Here's how the part is built. I have some questions about the finished solid (model axes, mm). Face numbers are marked on the shaded views. A direction names the side the tool comes from. Coordinates: 2 decimals unless noted, no trailing zeros. Loops run counter-clockwise (first coordinate to the right, second up) from the corner with the lowest first, then second, coordinate; pieces in that order, holes last. Notation, with made-up numbers: (-33.5, 43) -> (16.5, 43) arc R28 cw to (16.5, 75) -> close; hole circle Ø10 at (74.25, -0.5). An arc over 180 degrees is marked (long way). Answer as a JSON object with one key per item and string values. Group by question number.
Q1. I want a section at A-A on y = 3.5. Count the separate pieces of the cut face and the enclosed holes in it, then the cut area to 3 significant figures.
Q2. On a 3-axis mill with a long thin cutter (end or side, diameter ignored), from which of +Z, -Z, +X, -X, +Y, -Y can I reach the whole of each face in a straight line? I mean the marked faces 5, 6, 7 and 8. Say none if no direction works.
Q3. Thinking about a two-plate mould opening in Z: for the marked faces 1, 2, 3 and 4, which applies, released by +Z, released by -Z, zero draft, split by the parting line, or undercut?
Q4. I want a section at D-D on z = -9.5. Write out the boundary of the cut face in (x, y), then the cut area to 3 significant figures.
Q5. I need wall thicknesses on line 1 (X direction, y = 0.5, z = -13); line 2 (X direction, y = 1, z = -1.25); line 3 (Y direction, x = -3, z = 1). Which ranges of each line are inside material? Lowest first, please.
Q6. I'm going to push flat-ended pins straight in: pin 1 (2.5 mm diameter, centred on y = 5.5, z = -13, fed in from -X); pin 2 (1.5 mm diameter, centred on x = -10, z = -6, fed in from +Y); pin 3 (4 mm diameter, centred on y = 3, z = -14, fed in from +X). Where does each tip first touch, or does it pass through?
Q7. I want a section at B-B on z = -1.75. Write out the boundary of the cut face in (x, y), then the cut area to 3 significant figures.
Q8. I want a section at C-C on x = -12. Write out the boundary of the cut face in (y, z) (3 decimals).
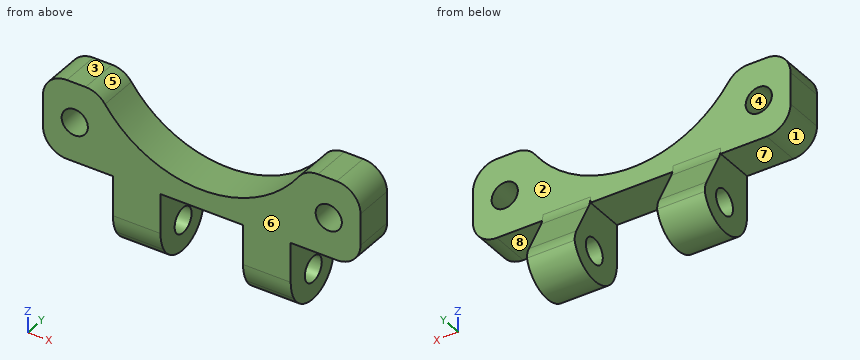
```python
from build123d import *

# Parameters (mm, degrees)
ESQUISSE1_W                    = 40
ESQUISSE1_H                    = 10
BOSS_EXTRU_1_DEPTH             = 5
ESQUISSE2_R                    = 1.65
ENL_V_MAT_EXTRU_1_DEPTH        = 5
BOSS_EXTRU_2_REACH             = 41.929
ESQUISSE3_W                    = 6
ESQUISSE3_H                    = 10
BOSS_EXTRU_2_DIRECTION_2_DEPTH = 5
ESQUISSE4_R                    = 1.6
ENL_V_MAT_EXTRU_2_DEPTH        = 38.217801601
CONG_1_R                       = 5
ENL_V_MAT_EXTRU_3_DEPTH        = 38.217801601
CONG_3_R                       = 3
CONG_4_R                       = 3
CONG_5_R                       = 3
ENL_V_MAT_EXTRU_4_REACH        = 44.982
CONG_6_R                       = 3
CONG_7_START                   = -30.067545716
CONG_7_DEPTH                   = 22.4


with BuildPart() as part:
    # Esquisse1 → Boss.-Extru.1 (new body)
    with BuildSketch(Plane(origin=(0, 0, 0), x_dir=(1, 0, 0), z_dir=(0, 1, 0))):
        with Locations((-18.867545716, 2.655728702)):
            Rectangle(ESQUISSE1_W, ESQUISSE1_H)
    extrude(amount=BOSS_EXTRU_1_DEPTH)

    # Esquisse2 → Enlèv. mat.-Extru.1 (cut)
    with BuildSketch(Plane(origin=(0, 5, 0), x_dir=(1, 0, 0), z_dir=(0, 1, 0))):
        with Locations(Location((-34.867545716, 2.655728702, 0), (0, 0, 270))):
            Circle(ESQUISSE2_R)
        with Locations(Location((-2.867545716, 2.655728702, 0), (0, 0, 270))):
            Circle(ESQUISSE2_R)
    extrude(amount=-ENL_V_MAT_EXTRU_1_DEPTH, mode=Mode.SUBTRACT)

    # Boss.-Extru.2: up to this face of the body (flat: up to its plane)
    boss_extru_2_end = Plane(part.part.faces().sort_by_distance((-18.867545716, 0, -2.655728702))[0])
    # Esquisse3 → Boss.-Extru.2 (add, up to the picked face)
    with BuildSketch(Plane(origin=(0, 5, 0), x_dir=(1, 0, 0), z_dir=(0, 1, 0)), mode=Mode.PRIVATE) as boss_extru_2_sk1:
        with Locations((-10.667545716, 12.655728702)):
            Rectangle(ESQUISSE3_W, ESQUISSE3_H)
    boss_extru_2_tool1 = split(extrude(boss_extru_2_sk1.sketch, amount=-BOSS_EXTRU_2_REACH, mode=Mode.PRIVATE), bisect_by=boss_extru_2_end, keep=Keep.BOTH, mode=Mode.PRIVATE)
    # Esquisse3 → Boss.-Extru.2 (add, up to the picked face)
    with BuildSketch(Plane(origin=(0, 5, 0), x_dir=(1, 0, 0), z_dir=(0, 1, 0)), mode=Mode.PRIVATE) as boss_extru_2_sk2:
        with Locations((-27.067545716, 12.655728702)):
            Rectangle(ESQUISSE3_W, ESQUISSE3_H)
    boss_extru_2_tool2 = split(extrude(boss_extru_2_sk2.sketch, amount=-BOSS_EXTRU_2_REACH, mode=Mode.PRIVATE), bisect_by=boss_extru_2_end, keep=Keep.BOTH, mode=Mode.PRIVATE)
    add(boss_extru_2_tool1.solids().sort_by(Axis((-10.667546, 5, -12.655729), (0, -1, 0)))[0])
    add(boss_extru_2_tool2.solids().sort_by(Axis((-27.067546, 5, -12.655729), (0, -1, 0)))[0])

    # Esquisse3 → Boss.-Extru.2 direction 2 (add)
    with BuildSketch(Plane(origin=(0, 5, 0), x_dir=(1, 0, 0), z_dir=(0, 1, 0))):
        with Locations((-10.667545716, 12.655728702)):
            Rectangle(ESQUISSE3_W, ESQUISSE3_H)
        with Locations((-27.067545716, 12.655728702)):
            Rectangle(ESQUISSE3_W, ESQUISSE3_H)
    extrude(amount=BOSS_EXTRU_2_DIRECTION_2_DEPTH)

    # Esquisse4 → Enlèv. mat.-Extru.2 (cut, through all)
    with BuildSketch(Plane(origin=(-7.667545716, 0, 0), x_dir=(0, 0, -1), z_dir=(1, 0, 0))):
        with Locations((13.380728702, 4.275)):
            Circle(ESQUISSE4_R)
    extrude(amount=-ENL_V_MAT_EXTRU_2_DEPTH, mode=Mode.SUBTRACT)

    # Congé1
    cong_1_edges = [part.edges().sort_by_distance(p)[0] for p in [
        (-27.067545716, 0, -17.655728702),
        (-10.667545716, 0, -17.655728702),
    ]]
    fillet(cong_1_edges, radius=CONG_1_R)

    # Esquisse5 → Enlèv. mat.-Extru.3 (cut, through all)
    with BuildSketch(Plane(origin=(-7.667545716, 0, 0), x_dir=(0, 0, -1), z_dir=(1, 0, 0))):
        Polygon((7.655728702, 5), (13.380728702, 8), (17.655728702, 8), (17.655728702, 10), (7.655728702, 10), align=None)
    extrude(amount=-ENL_V_MAT_EXTRU_3_DEPTH, mode=Mode.SUBTRACT)

    # Congé3
    cong_3_edges = [part.edges().sort_by_distance(p)[0] for p in [
        (-10.667545716, 8, -13.380728702),
        (-27.067545716, 8, -13.380728702),
    ]]
    fillet(cong_3_edges, radius=CONG_3_R)

    # Congé4
    cong_4_edges = [part.edges().sort_by_distance(p)[0] for p in [
        (-10.667545716, 5, -7.655728702),
        (-27.067545716, 5, -7.655728702),
    ]]
    fillet(cong_4_edges, radius=CONG_4_R)

    # Congé5
    cong_5_edges = [part.edges().sort_by_distance(p)[0] for p in [
        (-38.867545716, 2.5, -7.655728702),
        (-38.867545716, 2.5, 2.344271298),
        (1.132454284, 2.5, 2.344271298),
        (1.132454284, 2.5, -7.655728702),
    ]]
    fillet(cong_5_edges, radius=CONG_5_R)

    # Esquisse6 → Enlèv. mat.-Extru.4 (cut, up to next)
    with BuildSketch(Plane(origin=(0, 5, 0), x_dir=(1, 0, 0), z_dir=(0, 1, 0)), mode=Mode.PRIVATE) as enl_v_mat_extru_4_sk1:
        with BuildLine():
            Line((-31.867545716, -2.344271298), (-5.867545716, -2.344271298))
            ThreePointArc((-5.867545716, -2.344271298), (-18.867545716, 5.172413928), (-31.867545716, -2.344271298))
        make_face()
    enl_v_mat_extru_4_tool1 = extrude(enl_v_mat_extru_4_sk1.sketch, amount=-ENL_V_MAT_EXTRU_4_REACH, mode=Mode.PRIVATE) & part.part
    add(enl_v_mat_extru_4_tool1.solids().sort_by_distance((-18.867546, 5, -0.73807))[0], mode=Mode.SUBTRACT)

    # Congé6
    cong_6_edges = [part.edges().sort_by_distance(p)[0] for p in [
        (-31.867545716, 2.5, 2.344271298),
        (-5.867545716, 2.5, 2.344271298),
    ]]
    fillet(cong_6_edges, radius=CONG_6_R)

    # Congé7: read off the stored shape, not the designer's step
    # Congé7 outline → Congé7 (cut)
    with BuildSketch(Plane.YZ.offset(CONG_7_START)):
        with BuildLine():
            Line((8, -17.655728702), (8, -14.119135311))
            ThreePointArc((8, -14.119135311), (4.626068057, -17.103985452), (0.613789507, -15.055969837))
            ThreePointArc((0.613789507, -15.055969837), (2.450608472, -16.956961414), (5, -17.655728702))
            Line((5, -17.655728702), (8, -17.655728702))
        make_face()
    extrude(amount=CONG_7_DEPTH, mode=Mode.SUBTRACT)


solid = part.part
```
Result set:
{
 "1": {"separate pieces": "3", "enclosed holes": "2", "area": "315 mm²"},
 "2": {"face 5": "+Z, +Y, -Y", "face 6": "+Z, -Z, +X, -X, -Y", "face 7": "-Z, -X, +Y, -Y", "face 8": "-Z, +X, +Y, -Y"},
 "3": {"face 1": "released by -Z", "face 2": "zero draft", "face 3": "released by +Z", "face 4": "undercut"},
 "4": {"outline": "(-30.07, 0) -> (-24.07, 0) -> (-24.07, 5.97) -> (-30.07, 5.97) -> close; (-13.67, 0) -> (-7.67, 0) -> (-7.67, 5.97) -> (-13.67, 5.97) -> close", "area": "71.6 mm²"},
 "5": {"line 1": "x = -30.07 to -24.07, -13.67 to -7.67", "line 2": "x = -38.87 to -35.73, -34 to -28.98, -8.75 to -3.73, -2 to 1.13", "line 3": "y = 0 to 5"},
 "6": {"pin 1": "stops at x = -30.07", "pin 2": "stops at y = 5", "pin 3": "stops at x = -7.67"},
 "7": {"outline": "(-38.87, 0) -> (-36.25, 0) -> (-36.25, 5) -> (-38.87, 5) -> close; (-33.49, 0) -> (-28.4, 0) -> (-28.4, 5) -> (-33.49, 5) -> close; (-9.33, 0) -> (-4.25, 0) -> (-4.25, 5) -> (-9.33, 5) -> close; (-1.49, 0) -> (1.13, 0) -> (1.13, 5) -> (-1.49, 5) -> close", "area": "77.0 mm²"},
 "8": {"outline": "(0, -12.656) arc R5 ccw to (0.614, -15.056) arc R4 ccw to (8, -14.119) arc R3 ccw to (7.657, -12.727) -> (5.343, -8.31) arc R3 cw to (5, -6.917) -> (5, -3.508) -> (0, -3.508) -> close; hole circle Ø3.2 at (4.275, -13.381)"}
}
